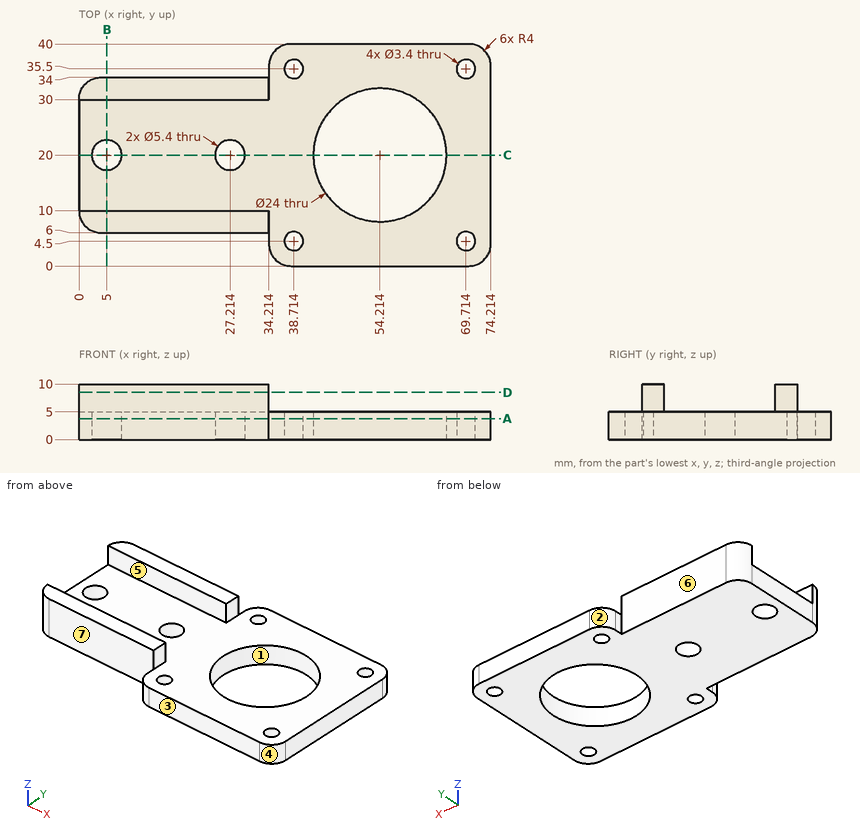
Geometry: see drawing. Coordinates: mm, zero at the bounding-box minimum. A direction names the side the tool comes from. Round coordinates to 2 decimals unless told otherwise and drop trailing zeros. Write each loop counter-clockwise with the first axis right and the second up, starting at its lowest first coordinate (ties: lowest second). Pieces come first, ordered by that corner, then holes. Notation, with made-up numbers: M 71.5,9 L 117.5,9 A16 ccw 117.5,20 Z; hole C 53.25,-4 d5. An arc over 180 degrees is marked long. Answer in a Markdown table with one row per item. Add a question column.
(1) Reachability of the marked faces 5, 6 and 7 from +Z, -Z, +X, -X, +Y, -Y: full face, straight path, thin tool, end or side. Return the list, or none.
(2) Draft query along X for the marked faces 1, 2, 3 and 4. Return one class per face: pulls with the +X half, pulls with the -X half, needs draft (parallel to the pull), parting line crosses it, or undercut.
(3) Cut plane A-A, the plane z = 3.75. Return the cut outline in (x, y), then the cut area to 3 significant figures.
(4) Cut plane B-B, the plane x = 5. Return the cut outline in (y, z), then the cut area to 3 significant figures.
(5) Cut plane D-D, the plane z = 8.5. Return the cut outline in (x, y), then the cut area to 3 significant figures.
(6) Cut plane C-C, the plane y = 20. Return the cut outline in (x, z), then the cut area to 3 significant figures.
(7) Contact query for flat-ended pins moving along their axis: pin 1 (2 mm diameter, centred on y = 7.5, z = 6.5, fed in from +X); pin 2 (3 mm diameter, centred on x = 13, z = 3.5, fed in from -Y); pin 3 (4 mm diameter, centred on x = 38.71, y = 35.5, fed in from +Z); pin 4 (4 mm diameter, centred on x = 49.5, y = 9.5, fed in from -Z). Output: stop coordinate, or through.
(8) Ray query, L1, parallel to Y at x = 27.5, z = 7.25; L2, parallel to Z at x = 57, y = 32; L3, parallel to Y at x = 5, z = 1.95. Return the intervals inside material, ascending.
Established:
| question | item | result |
|---|---|---|
| 1 | face 5 | +Z, +X, -X |
| 1 | face 6 | +Z, -Z, -X, +Y |
| 1 | face 7 | +Z, -Z, -X, -Y |
| 2 | face 1 | undercut |
| 2 | face 2 | pulls with the -X half |
| 2 | face 3 | needs draft |
| 2 | face 4 | pulls with the +X half |
| 3 | outline | M 0,10 A4 ccw 4,6 L 34.21,6 L 34.21,4 A4 ccw 38.21,0 L 70.21,0 A4 ccw 74.21,4 L 74.21,36 A4 ccw 70.21,40 L 38.21,40 A4 ccw 34.21,36 L 34.21,34 L 4,34 A4 ccw 0,30 Z; hole C 5,20 d5.4; hole C 27.21,20 d5.4; hole C 38.71,4.5 d3.4; hole C 38.71,35.5 d3.4; hole C 54.21,20 d24; hole C 69.71,4.5 d3.4; hole C 69.71,35.5 d3.4 |
| 3 | area | 2,000 mm² |
| 4 | outline | M 6,0 L 17.3,0 L 17.3,5 L 10,5 L 10,10 L 6,10 Z; M 22.7,0 L 34,0 L 34,10 L 30,10 L 30,5 L 22.7,5 Z |
| 4 | area | 153 mm² |
| 5 | outline | M 0,10 A4 ccw 4,6 L 34.21,6 L 34.21,10 Z; M 0,30 L 34.21,30 L 34.21,34 L 4,34 A4 ccw Z |
| 5 | area | 267 mm² |
| 6 | outline | M 0,0 L 2.3,0 L 2.3,5 L 0,5 Z; M 7.7,0 L 24.51,0 L 24.51,5 L 7.7,5 Z; M 29.91,0 L 42.21,0 L 42.21,5 L 29.91,5 Z; M 66.21,0 L 74.21,0 L 74.21,5 L 66.21,5 Z |
| 6 | area | 197 mm² |
| 7 | pin 1 | x = 34.21 |
| 7 | pin 2 | y = 6 |
| 7 | pin 3 | z = 5 |
| 7 | pin 4 | z = 0 |
| 8 | L1 | 6 to 10, 30 to 34 |
| 8 | L2 | 0 to 5 |
| 8 | L3 | 6 to 17.3, 22.7 to 34 |
